Solid Edge part; units mm, degrees
sketch "Sketch1" plane through (0, 0, 0) normal (0, 0, 1) x (1, 0, 0)
  line L0 (-4, -20) -> (4, -20)
  line L1 (4, -20) -> (4, 20)
  line L2 (4, 20) -> (-4, 20)
  line L3 (-4, 20) -> (-4, -20)
  dimension "D1" = 4
  dimension "D2" = 4
extrude "Protrusion1" add sketch "Sketch1" against normal blind 7
fillet "Round_4" radius 4 4 edges at (4, -20, -3.5) (-4, -20, -3.5) (4, 20, -3.5) (-4, 20, -3.5)
properties material "Stainless steel"
Geometry check sheet. Reference: the model listing, model coordinates, mm. Coordinates: 2 decimals unless noted, no trailing zeros. Order: outer loops, then holes, each group sorted by start corner. A loop starts at its lowest first (then second) coordinate and runs counter-clockwise, first axis right, second up. Notation, with made-up numbers: (31.5, -24) - (74.5, -24) arc R22 ccw to (74.5, 13) - close; hole circle Ø3 at (21.25, -37.5). An arc over 180 degrees is marked (long way). Answer as a JSON object with one key per item and string values. Group by question number.
Item 1: Sectioned sample at C-C, the plane x = 3.25. Record the cut outline in (y, z), and give its area (3 significant figures).
Item 2: Sectioned sample at B-B, the plane x = -1.75. Record the cut outline in (y, z).
Item 3: Depth check by flat-ended pin: pin 1 Ø1.5 at (x, z) = (0.5, -1.5) entering from +Y; pin 2 Ø1 at (x, z) = (3, -4.5) entering from -Y. Enter the tip coordinate at first touch or a pass-through.
Item 4: Scan lines: probe 1 along Y at (x, z) = (-1.75, -2); probe 2 along Y at (x, z) = (-0.5, -5); probe 3 along X at (y, z) = (18, -6.5). Record each from-to range of solid material in increasing order.
Resolved:
{
 "1": {"outline": "(-18.33, -7) - (18.33, -7) - (18.33, 0) - (-18.33, 0) - close", "area": "257 mm^2"},
 "2": {"outline": "(-19.6, -7) - (19.6, -7) - (19.6, 0) - (-19.6, 0) - close"},
 "3": {"pin 1": "y = 20", "pin 2": "y = -19.12"},
 "4": {"probe 1": "-19.6 to 19.6", "probe 2": "-19.97 to 19.97", "probe 3": "-3.46 to 3.46"}
}
